Work out the finished part from the listing and answer in its coordinate system (mm). A direction names the side the tool comes from. Round coordinates to 2 decimals unless told otherwise and drop trailing zeros. Write each loop counter-clockwise with the first axis right and the second up, starting at its lowest first coordinate (ties: lowest second). Pieces come first, ordered by that corner, then holes. Notation, with made-up numbers: (54, 70) - (64, 70) arc R15 ccw to (64, 99) - close; hole circle Ø11 at (19.25, 32.5). An arc over 180 degrees is marked (long way). Answer as a JSON object with one key per item and string values.
Autodesk Inventor part; units mm, degrees
ref_plane "YZ Plane" through (0, 0, 0) normal (1, 0, 0) x (0, 1, 0)
ref_plane "XZ Plane" through (0, 0, 0) normal (0, 1, 0) x (-1, 0, 0)
ref_plane "XY Plane" through (0, 0, 0) normal (0, 0, 1) x (1, 0, 0)
sketch "Sketch1" plane through (0, 0, 0) normal (0, 0, 1) x (1, 0, 0)
  line L0 (0, 0) -> (69.85, 0)
  line L1 (69.85, 0) -> (69.85, 114.3)
  line L2 (69.85, 114.3) -> (0, 114.3)
  line L3 (0, 114.3) -> (0, 0)
  circle A0 centre (34.925, 98.552) radius 2.5
  circle A1 centre (34.925, 15.748) radius 2.5
  circle A2 centre (34.925, 57.15) radius 3.75
  point P0 (34.925, 114.3)
  point P1 (0, 57.15)
  dimension "d0" = 69.85
  dimension "d1" = 114.3
  dimension "d13" = 82.804
  dimension "d14" = 5
  dimension "d15" = 5
  dimension "d16" = 7.5
  dimension "d17" = 15.748
extrude "Extrusion2" add sketch "Sketch1" along normal blind 12.7
sketch "Sketch3" plane through (0, 0, 0) normal (0, 0, -1) x (-1, 0, 0)
  line L0 (-67.31, 111.76) -> (-2.54, 111.76)
  line L1 (-2.54, 111.76) -> (-2.54, 2.54)
  line L2 (-2.54, 2.54) -> (-67.31, 2.54)
  line L3 (-67.31, 2.54) -> (-67.31, 111.76)
  circle A0 centre (-34.925, 57.15) radius 3.75
  circle A1 centre (-34.925, 15.748) radius 2.5
  circle A2 centre (-34.925, 98.552) radius 2.5
  line L4 (0, 0) -> (-69.85, 0)
  line L5 (0, 114.3) -> (0, 0)
  line L6 (-69.85, 114.3) -> (0, 114.3)
  line L7 (-69.85, 0) -> (-69.85, 114.3)
  dimension "d20" = 114.3
  dimension "d21" = 69.85
  dimension "d22" = 2.54
  dimension "d24" = 2.54
  dimension "d25" = 2.54
  dimension "d26" = 2.54
extrude "Extrusion3" cut sketch "Sketch3" against normal blind 10.16 contours L0 L1 L2 L3
sketch "Sketch4" plane through (0, 0, 10.16) normal (0, 0, -1) x (-1, 0, 0)
  circle A0 centre (-34.925, 57.15) radius 3.75
  circle A1 centre (-34.925, 98.552) radius 2.5
  circle A2 centre (-34.925, 15.748) radius 2.5
  line L0 (-67.31, 111.76) -> (-2.54, 111.76)
  line L1 (-67.31, 2.54) -> (-67.31, 111.76)
  line L2 (-2.54, 2.54) -> (-67.31, 2.54)
  line L3 (-2.54, 111.76) -> (-2.54, 2.54)
  circle A3 centre (-59.69, 104.14) radius 3.175
  circle A4 centre (-59.69, 104.14) radius 1.25
  circle A5 centre (-10.16, 104.14) radius 3.175
  circle A6 centre (-10.16, 104.14) radius 1.25
  circle A7 centre (-59.69, 10.16) radius 3.175
  circle A8 centre (-59.69, 10.16) radius 1.25
  circle A9 centre (-10.16, 10.16) radius 3.175
  circle A10 centre (-10.16, 10.16) radius 1.25
  point P0 (0, 0)
  dimension "d29" = 6.35
  dimension "d30" = 2.5
  dimension "d31" = 6.35
  dimension "d32" = 2.5
  dimension "d33" = 7.62
  dimension "d34" = 7.62
  dimension "d35" = 7.62
  dimension "d36" = 7.62
  dimension "d37" = 6.35
  dimension "d38" = 2.5
  dimension "d39" = 7.62
  dimension "d40" = 7.62
  dimension "d41" = 6.35
  dimension "d42" = 2.5
  dimension "d43" = 7.62
  dimension "d44" = 7.62
extrude "Extrusion4" add sketch "Sketch4" along normal blind 6.6 contours A3 | A5 | A7 | A9
fillet "Fillet1" radius 3.175 4 edges at (0, 57.15, 12.7) (69.85, 57.15, 12.7) (34.925, 114.3, 12.7) (34.925, 0, 12.7)
fillet "Fillet2" radius 3.175 8 edges at (0.9299, 113.3701, 11.7701) (0, 114.3, 4.7625) (68.9201, 113.3701, 11.7701) (69.85, 114.3, 4.7625) (0.9299, 0.9299, 11.7701) (0, 0, 4.7625) (68.9201, 0.9299, 11.7701) (69.85, 0, 4.7625)
equation "\"d17\" = -0.5 * d13 + 0.5 * d1"
equation "\"d24\" = d22"
equation "\"d25\" = d22"
equation "\"d26\" = d22"
equation "\"d31\" = d29"
equation "\"d32\" = d30"
equation "\"d34\" = d33"
equation "\"d35\" = d33"
equation "\"d36\" = d33"
equation "\"d37\" = d29"
equation "\"d38\" = d30"
equation "\"d39\" = d33"
equation "\"d40\" = d33"
equation "\"d41\" = d29"
equation "\"d42\" = d30"
equation "\"d43\" = d33"
equation "\"d44\" = d33"
properties part number "LightSwitchCover" material "Nylon 6/6"
Item 1: Each of these flat-tipped pins is pushed along its axis until it touches: P1, Ø6, axis at x = 58, y = 20, coming from the -Z side; P2, Ø7, axis at x = 60, y = 10.5, coming from the -Z side; P3, Ø3, axis at x = 34.925, y = 15.748, coming from the +Z side; P4, Ø3, axis at y = 75.5, z = 3, coming from the -X side. Where does it stop, or does it pass through?
Results found:
{"P1": "z = 10.16", "P2": "z = 3.56", "P3": "through", "P4": "x = 0"}
Item 2: A cutting plane is placed at B-B (y = 57.15). Write down the section's boundary in (x, z) (3 decimals).
Results found:
{"outline": "(0, 0) - (2.54, 0) - (2.54, 10.16) - (31.175, 10.16) - (31.175, 12.7) - (3.175, 12.7) arc R3.175 ccw to (0, 9.525) - close; (38.675, 10.16) - (67.31, 10.16) - (67.31, 0) - (69.85, 0) - (69.85, 9.525) arc R3.175 ccw to (66.675, 12.7) - (38.675, 12.7) - close"}
Item 3: A cutting plane is placed at A-A (z = 5). Give the number of separate pieces and of enclosed holes in the cut face, and give its area (3 significant figures).
Results found:
{"separate pieces": "5", "enclosed holes": "5", "area": "1,010 mm²"}
Item 4: Determine the mould class of faces 3 (the cylindrical face through (68.9, 113.39, 4.7)), 4 (the flat face through (0, 58, 5)), 5 (the flat face through (35, 111.76, 5)) for opening direction Y: pulls with the +Y half, pulls with the -Y half, needs draft (parallel to the pull), parting line crosses it, or undercut.
Results found:
{"face 3": "pulls with the +Y half", "face 4": "needs draft", "face 5": "undercut"}
Item 5: A cutting plane is placed at C-C (y = 71). Write down the section's boundary in (x, z) (3 decimals), and give its area (3 significant figures).
Results found:
{"outline": "(0, 0) - (2.54, 0) - (2.54, 10.16) - (67.31, 10.16) - (67.31, 0) - (69.85, 0) - (69.85, 9.525) arc R3.175 ccw to (66.675, 12.7) - (3.175, 12.7) arc R3.175 ccw to (0, 9.525) - close", "area": "225 mm²"}
Item 6: For faces 1 (the flat face through (1, 57, 0)), 2 (the cylindrical face through (60.611, 103.295, 6.906)), determine the directions among +Z, -Z, +X, -X, +Y, -Y from which every point of the face is accessible in a straight line to the end or side of a thin tool.
Results found:
{"face 1": "-Z, +X, -X, +Y, -Y", "face 2": "-Z"}
Item 7: Consider line 1 along Y through (x, z) = (59.69, 7) (3 decimals); line 2 along Y through (x, z) = (36, 2.25); line 3 along X through (y, z) = (7.5, 6). Determine where each line is inside the solid, lowest interval first.
Results found:
{"line 1": "0 to 2.54, 6.985 to 8.91, 11.41 to 13.335, 100.965 to 102.89, 105.39 to 107.315, 111.76 to 114.3", "line 2": "0 to 2.54, 111.76 to 114.3", "line 3": "0 to 2.54, 8.43 to 11.89, 57.96 to 61.42, 67.31 to 69.85"}
Item 8: A cutting plane is placed at D-D (x = 10.16). Write down the section's boundary in (y, z) (3 decimals).
Results found:
{"outline": "(0, 0) - (2.54, 0) - (2.54, 10.16) - (6.985, 10.16) - (6.985, 3.56) - (8.91, 3.56) - (8.91, 10.16) - (11.41, 10.16) - (11.41, 3.56) - (13.335, 3.56) - (13.335, 10.16) - (100.965, 10.16) - (100.965, 3.56) - (102.89, 3.56) - (102.89, 10.16) - (105.39, 10.16) - (105.39, 3.56) - (107.315, 3.56) - (107.315, 10.16) - (111.76, 10.16) - (111.76, 0) - (114.3, 0) - (114.3, 9.525) arc R3.175 ccw to (111.125, 12.7) - (3.175, 12.7) arc R3.175 ccw to (0, 9.525) - close"}
